The drawing under review shows one solid part. Ordinate dimensions are in mm from its lowest x, y, z. A direction names the side the tool comes from. Round coordinates to 2 decimals unless told otherwise and drop trailing zeros. Write each loop counter-clockwise with the first axis right and the second up, starting at its lowest first coordinate (ties: lowest second). Pieces come first, ordered by that corner, then holes. Notation, with made-up numbers: M 24,-12 L 39,-12 A10 ccw 39,-3 Z; hole C 31.5,45 d2. An arc over 180 degrees is marked long. One line per item, written item: value. Start each with the question number.
1) Take a section at C-C, the plane z = 10.5. Write out the cut boundary in (x, y).
2) Tool access review of the marked faces 4, 5 and 6: name each direction out of +Z, -Z, +X, -X, +Y, -Y from which nothing blocks a thin tool from reaching the whole face with its end or side.
3) Wall thickness on probe 1 along Y at (x, z) = (5.25, 10.5); probe 2 along X at (y, z) = (5.75, 15.25): over which ranges is each line inside the solid? List them lowest first.
4) Mouldability with a two-part tool opening along Y and no side actions: class the marked faces 1, 2 and 3 as +Y half, -Y half, draft (parallel to the pull), parting line (faces both ways), or undercut.
5) For P1, Ø3.5, axis at x = 8, z = 9.5, coming from the -Y side; P2, Ø1.5, axis at y = 7.5, z = 7.5, coming from the -X side; P3, Ø2.5, axis at y = 7.5, z = 10.5, coming from the +X side; P4, Ø3.5, axis at y = 5, z = 8, coming from the +X side, all flat-tipped, find the tip position at first contact; note any pin that passes through.
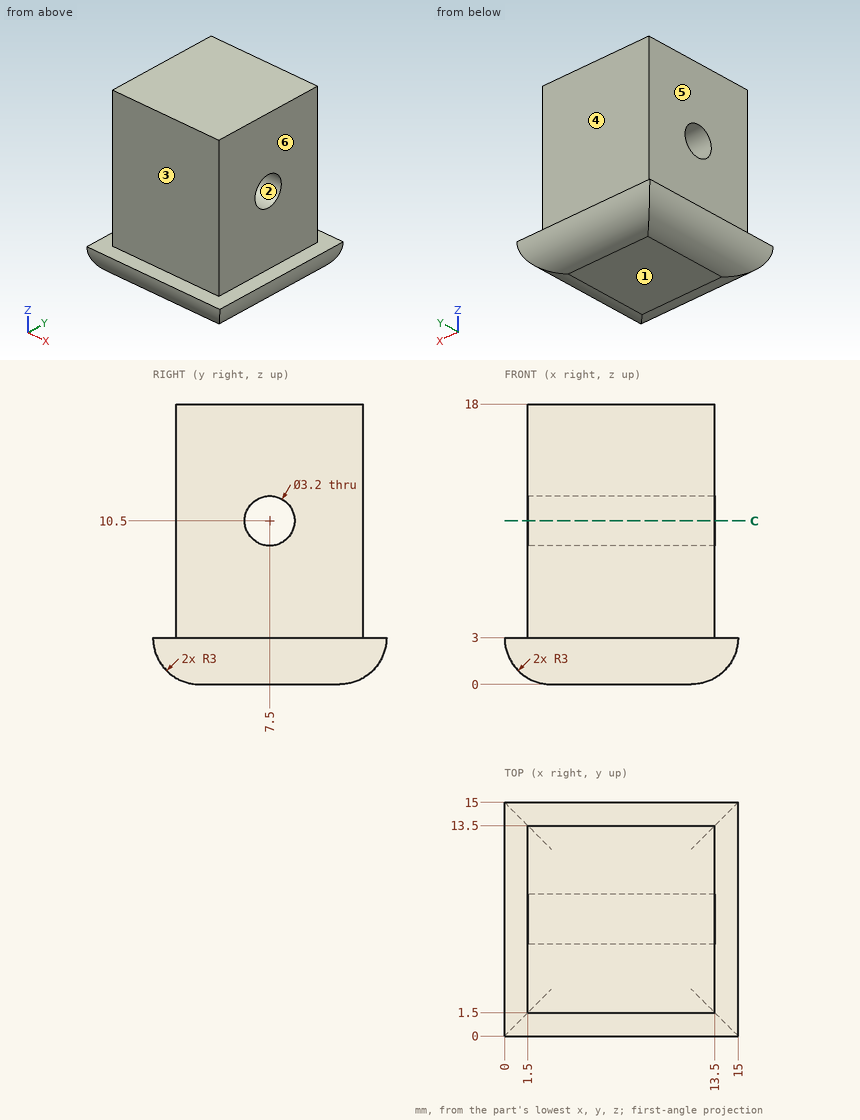
Checked values:
1. outline: M 1.5,1.5 L 13.5,1.5 L 13.5,5.9 L 1.5,5.9 Z; M 1.5,9.1 L 13.5,9.1 L 13.5,13.5 L 1.5,13.5 Z
2. face 4: +Z, +X, -X, +Y
2. face 5: +Z, -X, +Y, -Y
2. face 6: +Z, +X, +Y, -Y
3. probe 1: y = 1.5 to 5.9, 9.1 to 13.5
3. probe 2: x = 1.5 to 13.5
4. face 1: draft
4. face 2: undercut
4. face 3: -Y half
5. P1: stops at y = 1.5
5. P2: stops at x = 1.5
5. P3: passes through
5. P4: stops at x = 13.5
